Here's how the part is built. I have some questions about the finished solid (model axes, mm). A direction names the side the tool comes from. Give positions to 0.01 mm unless a question says otherwise; leave off trailing zeros. Loops run counter-clockwise (first coordinate to the right, second up) from the corner with the lowest first, then second, coordinate; pieces in that order, holes last. Notation, with made-up numbers: M 15.5,79 L 51.5,79 A19 ccw 51.5,110 Z; hole C 23.5,-13.5 d7. An arc over 180 degrees is marked long. Write item = value, one per line. Start each with the question number.
Autodesk Inventor part; units mm, degrees
ref_plane "YZ Plane" through (0, 0, 0) normal (1, 0, 0) x (0, 1, 0)
ref_plane "XZ Plane" through (0, 0, 0) normal (0, 1, 0) x (-1, 0, 0)
ref_plane "XY Plane" through (0, 0, 0) normal (0, 0, 1) x (1, 0, 0)
sketch "Sketch1" plane through (0, 0, 0) normal (0, 1, 0) x (-1, 0, 0)
  circle A0 centre (0, 0) radius 18.034
  dimension "d0" = 36.068
extrude "Extrusion1" add sketch "Sketch1" along normal blind 324.612
sketch "Sketch2" plane through (0, 324.612, 0) normal (0, 1, 0) x (1, 0, 0)
  circle A0 centre (0, 0) radius 9.525
  dimension "d3" = 19.05
extrude "Extrusion2" add sketch "Sketch2" along normal blind 25.4
sketch "Sketch3" plane through (0, 0, 0) normal (0, -1, 0) x (1, 0, 0)
  line L0 (-7.62, -10.16) -> (7.62, -10.16)
  line L1 (7.62, -10.16) -> (7.62, 10.16)
  line L2 (7.62, 10.16) -> (-7.62, 10.16)
  line L3 (-7.62, 10.16) -> (-7.62, -10.16)
  line L4 (-7.62, -10.16) -> (7.62, 10.16) construction
  line L5 (7.62, -10.16) -> (-7.62, 10.16) construction
  point P0 (0, 0)
  dimension "d6" = 15.24
  dimension "d7" = 20.32
extrude "Extrusion3" add sketch "Sketch3" along normal blind 18.288
sketch "Sketch4" plane through (7.62, 0, 10.16) normal (1, 0, 0) x (0, 0, -1)
  line L0 (0, 0) -> (20.32, 0)
  line L1 (20.32, 0) -> (20.32, -18.288)
  point P0 (10.16, 0)
  point P1 (10.16, -10.922)
  dimension "d10" = 10.922
  dimension "d11" = 10.16
hole "Hole1" at (7.62, -10.922, 0) direction (-1, 0, 0) diameter 6.35 end through all
sketch "Sketch5" plane through (7.62, 0, 10.16) normal (1, 0, 0) x (0, 0, -1)
  circle A0 centre (10.16, 340.614) radius 3.175
  line L0 (19.685, 350.012) -> (0.635, 350.012)
  point P0 (10.16, 0)
  dimension "d19" = 6.35
  dimension "d24" = 9.398
extrude "Extrusion4" cut sketch "Sketch5" along normal mid plane 127
properties part number "9 inch Linear Actuator"
Q1. We'd pull the mould along Z, two halves only. Please class faces 5 (the flat face through (0, -9, 10.16)), 6 (the flat face through (7.62, -7, 0)), 7 (the cylindrical face through (-0.107, -7.823, 0.688)): pulls with the +Z half, pulls with the -Z half, needs draft (parallel to the pull), parting line crosses it, or undercut.
Q2. If we section it at D-D, the plane z = -15: List the corners of the cut face in (x, y) for me.
Q3. On a 3-axis mill with a long thin cutter (end or side, diameter ignored), from which of +Z, -Z, +X, -X, +Y, -Y can I reach the whole of each face in a straight line? I mean faces 1 (the flat face through (0, -9, -10.16)), 2 (the flat face through (0, 350.012, 0)), 3 (the flat face through (-8, 324.612, -8)), 4 (the flat face through (-7.62, -7, 0)). Say none if no direction works.
Q4. If we section it at A-A, the plane z = 0: List the corners of the cut face in (x, y) for me (3 decimals).
Q5. If we section it at B-B, the plane x = 2.5: List the corners of the cut face in (y, z) for me (3 decimals).
Q6. Will these pins go through, and if not, where does the flat tip stop? pin 1 (12 mm diameter, centred on x = 6, y = 272.5, fed in from -Z); pin 2 (17 mm diameter, centred on x = 4, y = -7.5, fed in from +Z); pin 3 (5.5 mm diameter, centred on y = 340.614, z = 0, fed in from -X); pin 4 (20 mm diameter, centred on y = -9.5, z = -4.5, fed in from +X).
Q7. If we section it at C-C, the plane y = 289: List the corners of the cut face in (x, z) for me, then the cut area to 3 significant figures.
Q8. If I drill on line 1 along Y through (x, z) = (-1.25, 0); line 2 along Y through (x, z) = (-7, 12); line 3 along Y through (x, z) = (4, -1), over which ranges is the centre line in solid material (lowest first)?
Resolved:
q1.face_5 = pulls with the +Z half
q1.face_6 = needs draft
q1.face_7 = undercut
q2.outline = M -10.01,0 L 10.01,0 L 10.01,324.61 L -10.01,324.61 Z
q3.face_1 = -Z, +X, -X, -Y
q3.face_2 = +Z, -Z, +X, -X, +Y
q3.face_3 = +Y
q3.face_4 = +Z, -Z, -X, -Y
q4.outline = M -18.034,0 L -7.62,0 L -7.62,-7.747 L 7.62,-7.747 L 7.62,0 L 18.034,0 L 18.034,324.612 L 9.525,324.612 L 9.525,337.439 L -9.525,337.439 L -9.525,324.612 L -18.034,324.612 Z; M -9.525,343.789 L 9.525,343.789 L 9.525,350.012 L -9.525,350.012 Z; M -7.62,-18.288 L 7.62,-18.288 L 7.62,-14.097 L -7.62,-14.097 Z
q5.outline = M -18.288,-10.16 L 0,-10.16 L 0,-17.86 L 324.612,-17.86 L 324.612,-9.191 L 350.012,-9.191 L 350.012,9.191 L 324.612,9.191 L 324.612,17.86 L 0,17.86 L 0,10.16 L -18.288,10.16 Z; hole C -10.922,0 d6.35; hole C 340.614,0 d6.35
q6.pin_1 = -18.03
q6.pin_2 = 18.03
q6.pin_3 = through
q6.pin_4 = 17.98
q7.outline = C 0,0 d36.07
q7.area = 1,020 mm²
q8.line_1 = -18.29 to -14.1, -7.75 to 337.44, 343.79 to 350.01
q8.line_2 = 0 to 324.61
q8.line_3 = -18.29 to -13.94, -7.91 to 337.6, 343.63 to 350.01
